Autodesk Inventor part; units mm, degrees
ref_plane "WorkPlane11" through (0, 0, 0) normal (0, 0, 1) x (1, 0, 0)
ref_plane "Work Plane2" through (0, 0, -5.7) normal (0, 0, 1) x (1, 0, 0)
ref_plane "WorkPlane9" through (0, 0, 8.3) normal (0, 0, 1) x (1, 0, 0)
ref_plane "WorkPlane11" through (0, 0, 0) normal (0, 0, 1) x (1, 0, 0)
ref_plane "Work Plane2" through (0, 0, -5.7) normal (0, 0, 1) x (1, 0, 0)
ref_plane "WorkPlane9" through (0, 0, 8.3) normal (0, 0, 1) x (1, 0, 0)
sketch "Sketch1" plane through (0, 0, 0) normal (0, 0, 1) x (1, 0, 0)
  point P0 (0, 0)
sketch "Sketch2" plane through (0, 0, 0) normal (0, 0, 1) x (1, 0, 0)
  circle A0 centre (0, 0) radius 2.75
  dimension "d2" = 5.5
extrude "Extrusion1" add sketch "Sketch2" against normal blind 0.75
sketch "Sketch3" plane through (0, 0, -0.75) normal (0, 0, -1) x (-1, 0, 0)
  circle A0 centre (0, 0) radius 3
  circle A1 centre (0, 0) radius 2.75 construction
  dimension "d8" = 6
extrude "Extrusion2" add sketch "Sketch3" along normal blind 5.95
sketch "Sketch4" plane through (0, 0, 0) normal (0, 0, 1) x (1, 0, 0)
  circle A0 centre (0, 0) radius 5.65
  circle A1 centre (0, 0) radius 2.75 construction
  dimension "d12" = 11.3
extrude "Extrusion3" add sketch "Sketch4" along normal blind 3.3
sketch "Sketch5" plane through (0, 0, 0) normal (0, 1, 0) x (-1, 0, 0)
  line L0 (5.65, 0) -> (2.75, 0)
  line L1 (5.65, 2.9) -> (5.65, 0)
  line L2 (2.75, 0) -> (5.65, 2.9)
  line L3 (-5.65, 0) -> (5.65, 0) construction
  line L4 (0, -7.6493) -> (0, 5.8993)
  line L5 (0, -10.359) -> (0, 8.609)
  line L6 (5.65, 0) -> (5.65, 3.3)
  line L7 (-4.75, 0) -> (4.75, 0)
  line L8 (2.75, 0) -> (2.75, -0.75)
  dimension "d17" = 45
revolve "Revolution1" cut sketch "Sketch5" angle 360 about axis through (0, 0, -7.6493) along (0, 0, 1)
sketch "Sketch6" plane through (0, 0, 0) normal (0, 1, 0) x (-1, 0, 0)
  line L0 (0, 3.3) -> (0, 4.7133)
  line L1 (0, 3.3) -> (5.65, 3.3)
  arc A0 (5.65, 3.3) -> (0, 4.7133) centre (0, -7.2867) ccw
  line L2 (-5.65, 3.3) -> (5.65, 3.3) construction
  line L3 (0, -7.6493) -> (0, 5.8993)
  line L4 (0, -10.359) -> (0, 8.609)
  line L5 (5.65, 2.9) -> (5.65, 3.3)
  arc A1 (0, 4.7133) -> (-5.65, 3.3) centre (0, -7.2867) ccw
  dimension "d20" = 12
  dimension "d24" = 5.65
revolve "Revolution2" add sketch "Sketch6" angle 360 about axis through (0, 0, -7.6493) along (0, 0, 1)
fillet "Fillet1" radius 1.5 2 edges at (0, 2.75, 0) (0, -2.75, 0)
chamfer "Chamfer1" distance 1.25 distance2 0.25 1 edges at (3, 0, -0.75) measured on face at (-2.9612, -0.4812, -4.7167)
sketch "Sketch8" plane through (0, 0, 0) normal (0, 1, 0) x (-1, 0, 0)
  line L0 (-5.65, 4.7133) -> (5.65, 4.7133)
  line L1 (5.65, 4.7133) -> (5.65, 2.3133)
  line L2 (5.65, 2.3133) -> (-5.65, 2.3133)
  line L3 (-5.65, 2.3133) -> (-5.65, 4.7133)
  arc A0 (5.65, 3.3) -> (-5.65, 3.3) centre (0, -7.2867) ccw
  line L4 (-5.65, 2.9) -> (-5.65, 3.3)
  line L5 (5.65, 2.9) -> (5.65, 3.3)
  dimension "msp_d31" = 2.4
extrude "Extrusion4" cut sketch "Sketch8" against normal mid plane 1.6
thread "Thread1"
ref_plane "MSC_PF1" through (0, 0, 0) normal (1, 0, 0) x (0, 1, 0)
ref_plane "MSC_PT1" through (-5.65, 0, 2.9) normal (0, 0, -1) x (-1, 0, 0)
equation "\"d28\" = r"
equation "\"d29\" = msp_x"
equation "\"d30\" = 0.25 * PTC"
equation "\"d3\" = -msp_x + ParA"
equation "\"d8\" = NND"
equation "\"d9\" = msp_x - ParK + NLG - ParA"
equation "\"d12\" = Dk"
equation "\"d13\" = ParK"
equation "\"msp_d31\" = ParT"
equation "\"msp_d32\" = ParN"
equation "\"d2\" = 0.5 * PTC + msp_mdtds"
equation "\"d20\" = rf"
equation "\"d24\" = 0.5 * Dk"
equation "\"PTC\" = 1"
equation "\"NND\" = 6"
equation "\"msp_x\" = 1.25 * PTC"
equation "\"NLG\" = 10"
equation "\"msp_mdtds\" = NND - PTC"
equation "\"ParK\" = 3.3"
equation "\"ParN\" = 1.6"
equation "\"ParT\" = 2.4"
equation "\"r\" = 1.5"
equation "\"prf_c\" = 0"
equation "\"ParA\" = 2"
equation "\"Dk\" = 11.3"
equation "\"rf\" = 12"
equation "\"ParF\" = 1.4"
equation "\"THREADDIA\" = NND"
equation "\"PG\" = 1.2345"
equation "\"TEMPLATE\" = 1.2345"
properties part number "ISO 2010 - M6x10" material "Stainless Steel, 440C"
For this review, take the finished solid that the model builds, in its own axes (mm). A direction names the side the tool comes from. Give positions to 0.01 mm unless a question says otherwise; leave off trailing zeros. Write each loop counter-clockwise with the first axis right and the second up, starting at its lowest first coordinate (ties: lowest second). Pieces come first, ordered by that corner, then holes.
Item 1: Machinability: for faces 1 (the face through (3, 0, -4)), 2 (the face through (-0.11, 5.65, 3.1)), 3 (the face through (0, 0.8, 3)), which of the approach directions +Z, -Z, +X, -X, +Y, -Y give a long, thin tool a straight path to every point of the face, cutting with its end or side? Answer none if there is none.
Item 2: Insertion check: P1, Ø2.5, axis at x = -2.5, z = 4, coming from the +Y side; P2, Ø2.5, axis at x = 2, z = 3.5, coming from the -Y side; P3, Ø6, axis at y = -1, z = -4, coming from the -X side. Each pin has a flat end and moves straight along its axis. Give the tip position at first contact, or say it passes through.
Item 3: Take a section at B-B (z = -4.25). Give the boundary of the cut face in (x, y).
Item 4: Wall thickness on probe 1 along Z at (x, y) = (-1.5, -0.25); probe 2 along Y at (x, z) = (1.5, 3.25); probe 3 along Y at (x, z) = (3.25, 3): over which ranges is each line inside the solid? List them lowest first.
Item 5: Take a section at A-A (z = 1). Give the boundary of the cut face in (x, y), and give its area (3 significant figures).
Established:
1. face 1: -Z
1. face 2: +Z, -Z, +Y
1. face 3: +Z, +X, -X
2. P1: stops at y = 5.46
2. P2: stops at y = -5.6
2. P3: stops at x = -3
3. outline: circle Ø6 at (0, 0)
4. probe 1: z = -6.7 to 2.31
4. probe 2: y = -5.45 to -0.8, 0.8 to 5.45
4. probe 3: y = -4.62 to -0.8, 0.8 to 4.62
5. outline: circle Ø7.5 at (0, 0)
5. area: 44.2 mm2
